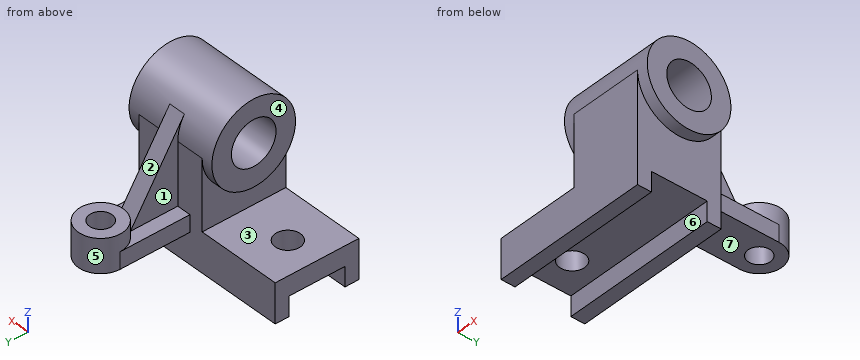
```python
from build123d import *

# Parameters (mm, degrees)
SKETCH1_W                = 112
SKETCH1_H                = 60
BOSS_EXTRUDE1_DEPTH      = 28
SKETCH2_W                = 14
SKETCH2_H                = 40
CUT_EXTRUDE1_DEPTH       = 120.28118041
SKETCH3_W                = 52
SKETCH3_H                = 60
BOSS_EXTRUDE2_DEPTH      = 50
BOSS_EXTRUDE3_DEPTH      = 8
BOSS_EXTRUDE3_DEPTH_BACK = 60
SKETCH4_R                = 30
SKETCH4_R_2              = 16
SKETCH5_R                = 16
CUT_EXTRUDE2_DEPTH       = 105.403065089
SKETCH6_W                = 32
SKETCH6_H                = 12
BOSS_EXTRUDE4_DEPTH      = 50
BOSS_EXTRUDE5_DEPTH      = 12
BOSS_EXTRUDE5_DEPTH_BACK = 12
SKETCH8_R                = 16
SKETCH8_R_2              = 8
SKETCH9_R                = 8
CUT_EXTRUDE3_DEPTH       = 138.069325525
RIB1_REACH               = 153.697
SKETCH17_WALL_W          = 377.032111856
SKETCH17_WALL_H          = 12
SKETCH18_R               = 9
CUT_EXTRUDE4_DEPTH       = 141.399430198


with BuildPart() as part:
    # Sketch1 → Boss-Extrude1 (new body)
    with BuildSketch(Plane.XY):
        Rectangle(SKETCH1_W, SKETCH1_H)
    extrude(amount=-BOSS_EXTRUDE1_DEPTH)

    # Sketch2 → Cut-Extrude1 (cut, through all)
    with BuildSketch(Plane(origin=(56, 0, 0), x_dir=(0, 0, -1), z_dir=(1, 0, 0))):
        with Locations((21, 0)):
            Rectangle(SKETCH2_W, SKETCH2_H)
    extrude(amount=-CUT_EXTRUDE1_DEPTH, mode=Mode.SUBTRACT)

    # Sketch3 → Boss-Extrude2 (add)
    with BuildSketch(Plane.XY):
        with Locations((30, 0)):
            Rectangle(SKETCH3_W, SKETCH3_H)
    extrude(amount=BOSS_EXTRUDE2_DEPTH)

    # Sketch4 → Boss-Extrude3 (add, two sides: drawn at the far end of the back side and taken through both)
    with BuildSketch(Plane.ZY.offset(-4).offset(-BOSS_EXTRUDE3_DEPTH_BACK)):
        with Locations((50, 0)):
            Circle(SKETCH4_R)
        with Locations((50, 0)):
            Circle(SKETCH4_R_2, mode=Mode.SUBTRACT)
    extrude(amount=BOSS_EXTRUDE3_DEPTH + BOSS_EXTRUDE3_DEPTH_BACK)

    # Sketch5 → Cut-Extrude2 (cut, through all)
    with BuildSketch(Plane.ZY.offset(-4)):
        with Locations((50, 0)):
            Circle(SKETCH5_R)
    extrude(amount=-CUT_EXTRUDE2_DEPTH, mode=Mode.SUBTRACT)

    # Sketch6 → Boss-Extrude4 (add)
    with BuildSketch(Plane(origin=(0, 30, 0), x_dir=(1, 0, 0), z_dir=(0, 1, 0))):
        with Locations((30, 0)):
            Rectangle(SKETCH6_W, SKETCH6_H)
    extrude(amount=BOSS_EXTRUDE4_DEPTH)

    # Sketch8 → Boss-Extrude5 (add, two sides: drawn at the far end of the back side and taken through both)
    with BuildSketch(Plane.XY.offset(6).offset(-BOSS_EXTRUDE5_DEPTH_BACK)):
        with Locations((30, 80)):
            Circle(SKETCH8_R)
        with Locations((30, 80)):
            Circle(SKETCH8_R_2, mode=Mode.SUBTRACT)
    extrude(amount=BOSS_EXTRUDE5_DEPTH + BOSS_EXTRUDE5_DEPTH_BACK)

    # Sketch9 → Cut-Extrude3 (cut, through all)
    with BuildSketch(Plane.XY.offset(6)):
        with Locations((30, 80)):
            Circle(SKETCH9_R)
    extrude(amount=-CUT_EXTRUDE3_DEPTH, mode=Mode.SUBTRACT)

    # Sketch17 wall → Rib1 (add, up to next)
    with BuildSketch(Plane(origin=(30, 44.612908816, 36.118776459), x_dir=(0, -0.541251763971, 0.84086058773), z_dir=(0, -0.84086058773, -0.541251763971)), mode=Mode.PRIVATE) as rib1_sk1:
        Rectangle(SKETCH17_WALL_W, SKETCH17_WALL_H)
    rib1_tool1 = extrude(rib1_sk1.sketch, amount=RIB1_REACH, mode=Mode.PRIVATE) - part.part
    add(rib1_tool1.solids().sort_by_distance((30, 44.612908816, 36.118776459))[0])

    # Sketch18 → Cut-Extrude4 (cut, through all)
    with BuildSketch(Plane.XY):
        with Locations((-32, 0)):
            Circle(SKETCH18_R)
    extrude(amount=-CUT_EXTRUDE4_DEPTH, mode=Mode.SUBTRACT)


solid = part.part
```
Input: part model. Units: mm. Frame: model coordinates. Face numbers are marked on the shaded views. A direction names the side the tool comes from. Coordinates: 2 decimals unless noted, no trailing zeros. Write each loop counter-clockwise with the first axis right and the second up, starting at its lowest first coordinate (ties: lowest second). Pieces come first, ordered by that corner, then holes.
1) Material intervals for line 1 along Y through (x, z) = (-32, -9.75); line 2 along Y through (x, z) = (30, 1.25); line 3 along X through (y, z) = (30.5, 11), sorted ascending.
2) Section C-C on x = -32. Output: boundary loops of the cut face in (y, z).
3) Section D-D on x = -48. Output: boundary loops of the cut face in (y, z), and give its area (3 significant figures).
4) Set-up query: the marked faces 4, 5, 6 and 7. Return all of +Z, -Z, +X, -X, +Y, -Y with unobstructed straight access to the full face (end or side cutting, diameter ignored); none if empty.
5) Section B-B on y = 0. Output: boundary loops of the cut face in (x, z).
6) Mould query, pull axis Z, two halves, no side actions, for the marked faces 1, 2 and 3. Classes: pulls with the +Z half, pulls with the -Z half, needs draft (parallel to the pull), parting line crosses it, or undercut.
7) Section A-A on z = -17. Output: boundary loops of the cut face in (x, y).
8) Pin query (flat end, axial travel): pin 1 Ø16 at (x, y) = (25.5, 80.5) entering from +Z; pin 2 Ø12 at (y, z) = (44, 11) entering from +X; pin 3 Ø11 at (x, z) = (-5, -18) entering from +Y. Return the tip coordinate at first contact, or that it passes through.
Check result:
1. line 1: y = -30 to -9, 9 to 30
1. line 2: y = -30 to 72, 88 to 96
1. line 3: x = 24 to 36
2. outline: (-30, -28) - (-20, -28) - (-20, -14) - (-9, -14) - (-9, 0) - (-30, 0) - close; (9, -14) - (20, -14) - (20, -28) - (30, -28) - (30, 0) - (9, 0) - close
3. outline: (-30, -28) - (-20, -28) - (-20, -14) - (20, -14) - (20, -28) - (30, -28) - (30, 0) - (-30, 0) - close
3. area: 1,120 mm2
4. face 4: +Z, -X, +Y, -Y
4. face 5: +Z
4. face 6: -Z, +X, -X
4. face 7: -Z, +X, -X, +Y
5. outline: (-56, -14) - (-41, -14) - (-41, 0) - (-56, 0) - close; (-23, -14) - (56, -14) - (56, 20) - (64, 20) - (64, 34) - (-4, 34) - (-4, 20) - (4, 20) - (4, 0) - (-23, 0) - close; (-4, 66) - (64, 66) - (64, 80) - (-4, 80) - close
6. face 1: needs draft
6. face 2: pulls with the +Z half
6. face 3: undercut
7. outline: (-56, -30) - (56, -30) - (56, -20) - (-56, -20) - close; (-56, 20) - (56, 20) - (56, 30) - (-56, 30) - close
8. pin 1: stops at z = 18
8. pin 2: stops at x = 46
8. pin 3: stops at y = 30
